from build123d import *

# Parameters (mm, degrees)
SKETCH2_R           = 6.35
BOSS_EXTRUDE1_DEPTH = 76.2
SKETCH3_W           = 12.7
SKETCH3_H           = 152.4
BOSS_EXTRUDE2_DEPTH = 12.7
BOSS_EXTRUDE3_DEPTH = 12.7
SKETCH6_W           = 12.7
SKETCH6_H           = 152.4
BOSS_EXTRUDE4_DEPTH = 12.7
BOSS_EXTRUDE5_DEPTH = 12.7
SKETCH8_W           = 19.05
SKETCH8_H           = 19.05
BOSS_EXTRUDE6_DEPTH = 101.6
SKETCH9_W           = 76.2
SKETCH9_H           = 29.319846112
CUT_EXTRUDE1_DEPTH  = 198.12
CUT_EXTRUDE2_DEPTH  = 102.6


with BuildPart() as part:
    # Sketch2 → Boss-Extrude1 (new body)
    with BuildSketch(Plane.XY):
        Circle(SKETCH2_R)
    extrude(amount=BOSS_EXTRUDE1_DEPTH)

    # Sketch3 → Boss-Extrude2 (add)
    with BuildSketch(Plane.XY.offset(76.2)):
        with Locations((0, -76.2)):
            Rectangle(SKETCH3_W, SKETCH3_H)
    extrude(amount=BOSS_EXTRUDE2_DEPTH)

    # Sketch4 → Boss-Extrude3 (add)
    with BuildSketch(Plane.XY.offset(76.2)):
        with BuildLine():
            Line((-6.35, 0), (6.35, 0))
            ThreePointArc((6.35, 0), (0, 6.35), (-6.35, 0))
        make_face()
    extrude(amount=BOSS_EXTRUDE3_DEPTH)

    # Sketch6 → Boss-Extrude4 (add)
    with BuildSketch(Plane(origin=(0, 0, 0), x_dir=(-1, 0, 0), z_dir=(0, 0, -1))):
        with Locations((0, -76.2)):
            Rectangle(SKETCH6_W, SKETCH6_H)
    extrude(amount=BOSS_EXTRUDE4_DEPTH)

    # Sketch7 → Boss-Extrude5 (add)
    with BuildSketch(Plane(origin=(0, 0, 0), x_dir=(-1, 0, 0), z_dir=(0, 0, -1))):
        with BuildLine():
            Line((-6.35, 0), (6.35, 0))
            ThreePointArc((6.35, 0), (0, 6.35), (-6.35, 0))
        make_face()
    extrude(amount=BOSS_EXTRUDE5_DEPTH)

    # Sketch8 → Boss-Extrude6 (add)
    with BuildSketch(Plane(origin=(0, 0, -12.7), x_dir=(-1, 0, 0), z_dir=(0, 0, -1))):
        with Locations((0, -152.4)):
            Rectangle(SKETCH8_W, SKETCH8_H)
    extrude(amount=-BOSS_EXTRUDE6_DEPTH)

    # Sketch9 → Cut-Extrude1 (cut)
    with BuildSketch(Plane(origin=(9.525, 0, 0), x_dir=(0, 0, -1), z_dir=(1, 0, 0))):
        with Locations((-38.1, -157.534923056)):
            Rectangle(SKETCH9_W, SKETCH9_H)
    extrude(amount=-CUT_EXTRUDE1_DEPTH, mode=Mode.SUBTRACT)

    # Sketch10 → Cut-Extrude2 (cut, through all)
    with BuildSketch(Plane.XY.offset(88.9)):
        with BuildLine():
            ThreePointArc((6.35, -152.4), (0, -146.05), (-6.35, -152.4))
            Line((-6.35, -152.4), (6.35, -152.4))
        make_face()
        with BuildLine():
            Line((6.35, -152.4), (-6.35, -152.4))
            ThreePointArc((-6.35, -152.4), (0, -158.75), (6.35, -152.4))
        make_face()
    extrude(amount=-CUT_EXTRUDE2_DEPTH, mode=Mode.SUBTRACT)


solid = part.part
Design review of the part built by this model. Coordinates are the model's own, in mm. A direction names the side the tool comes from. Coordinates: 2 decimals unless noted, no trailing zeros. Order: outer loops, then holes, each group sorted by start corner. A loop starts at its lowest first (then second) coordinate and runs counter-clockwise, first axis right, second up.
Item 1: For line 1 (Z direction, x = -2, y = -80); line 2 (Y direction, x = 0, z = -2.75) (3 decimals); line 3 (X direction, y = -152, z = 79) (3 decimals), list the stretches that pass through material, from the lowest coordinate up.
Item 2: Take a section at D-D, the plane z = 81. Write out the cut boundary in (x, y) (3 decimals).
Item 3: Take a section at C-C, the plane y = -88.5. Write out the cut boundary in (x, z), then the cut area to 3 significant figures.
Item 4: For pin 1 Ø10 at (y, z) = (-59, -7.5) entering from -X; pin 2 Ø4 at (y, z) = (-54.5, 80) entering from +X; pin 3 Ø1.6 at (x, z) = (-8, -4) entering from +Y (3 decimals), all flat-tipped, find the tip position at first contact; note any pin that passes through.
Item 5: Take a section at A-A, the plane x = 0. Write out the cut boundary in (y, z) (3 decimals), then the cut area to 3 significant figures.
Item 6: Take a section at B-B, the plane y = -152.4. Write out the cut boundary in (x, z) (3 decimals).
Item 7: The part is to be moulded in two halves that separate along X. For faces 1 (the cylindrical face through (1.38, -146.2, -6.26)), 2 (the flat face through (8, -142.875, -6)), 3 (the flat face through (-9.525, -153, -6)), say which applies: pulls with the +X half, pulls with the -X half, needs draft (parallel to the pull), parting line crosses it, or undercut.
Item 8: For faces 4 (the flat face through (0, -161.925, 82)), 5 (the flat face through (6.35, -72, 82)), 6 (the flat face through (-6.35, -72, -6)), list the 3-axis set-ups (+Z, -Z, +X, -X, +Y, -Y) from which the entire face can be reached by the end or side of a thin tool; tool diameter is ignored.
The answers:
1. line 1: z = -12.7 to 0, 76.2 to 88.9
1. line 2: y = -161.925 to -158.75, -146.05 to 6.35
1. line 3: x = -9.525 to -6.337, 6.337 to 9.525
2. outline: (-9.525, -161.925) - (9.525, -161.925) - (9.525, -142.875) - (6.35, -142.875) - (6.35, 0) arc R6.35 ccw to (-6.35, 0) - (-6.35, -142.875) - (-9.525, -142.875) - close; hole circle Ø12.7 at (0, -152.4)
3. outline: (-6.35, -12.7) - (6.35, -12.7) - (6.35, 0) - (-6.35, 0) - close; (-6.35, 76.2) - (6.35, 76.2) - (6.35, 88.9) - (-6.35, 88.9) - close
3. area: 323 mm2
4. pin 1: stops at x = -6.35
4. pin 2: stops at x = 6.35
4. pin 3: stops at y = -142.875
5. outline: (-161.925, -12.7) - (-158.75, -12.7) - (-158.75, 0) - (-161.925, 0) - close; (-161.925, 76.2) - (-158.75, 76.2) - (-158.75, 88.9) - (-161.925, 88.9) - close; (-146.05, -12.7) - (6.35, -12.7) - (6.35, 88.9) - (-146.05, 88.9) - (-146.05, 76.2) - (-6.35, 76.2) - (-6.35, 0) - (-146.05, 0) - close
5. area: 4,920 mm2
6. outline: (-9.525, -12.7) - (-6.35, -12.7) - (-6.35, 0) - (-9.525, 0) - close; (-9.525, 76.2) - (-6.35, 76.2) - (-6.35, 88.9) - (-9.525, 88.9) - close; (6.35, -12.7) - (9.525, -12.7) - (9.525, 0) - (6.35, 0) - close; (6.35, 76.2) - (9.525, 76.2) - (9.525, 88.9) - (6.35, 88.9) - close
7. face 1: undercut
7. face 2: needs draft
7. face 3: pulls with the -X half
8. face 4: +Z, -Z, +X, -X, -Y
8. face 5: +Z, -Z, +X, +Y
8. face 6: +Z, -Z, -X, +Y
